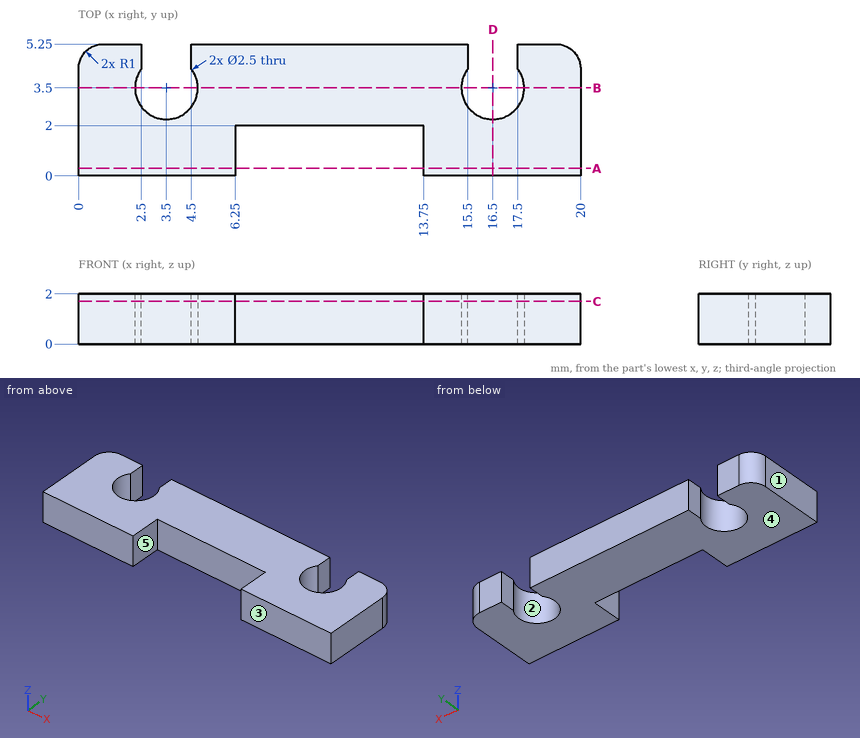
Answer from the drawing. Dimensions are ordinates in mm from the lowest x, y and z of the part. A direction names the side the tool comes from. Round coordinates to 2 decimals unless told otherwise and drop trailing zeros. Order: outer loops, then holes, each group sorted by start corner. A loop starts at its lowest first (then second) coordinate and runs counter-clockwise, first axis right, second up.
1) For the marked faces 4 and 5, determine the directions among +Z, -Z, +X, -X, +Y, -Y from which every point of the face is accessible in a straight line to the end or side of a thin tool.
2) The part is cut by section D-D on x = 16.5. Write down the section's boundary in (y, z).
3) The part is cut by section C-C on z = 1.7. Write down the section's boundary in (x, y).
4) Flat-ended cylindrical pins translate along their axes: pin 1 (0.5 mm diameter, centred on y = 5, z = 0.5, fed in from +X); pin 2 (1.1 mm diameter, centred on y = 5, z = 0.5, fed in from -X). Find the tip coordinate at first contact, or state that the pin passes through.
5) The mould has two halves that part along Y. Classify the marked faces 1, 2 and 3: released by +Y, released by -Y, zero draft, split by the parting line, or undercut.
6) Straight lines are drawn through the part: L1, parallel to X at y = 3.5, z = 1.1; L2, parallel to X at y = 0.3, z = 1; L3, parallel to X at y = 2.5, z = 0.1. For each, find the intervals that lie inside material, in ascending order.
7) The part is cut by section B-B on y = 3.5. Write down the section's boundary in (x, z).
8) The part is cut by section A-A on y = 0.3. Write down the section's boundary in (x, z).
Resolved:
1. face 4: -Z, +X, -X, +Y, -Y
1. face 5: +Z, -Z, -Y
2. outline: (0, 0) - (2.25, 0) - (2.25, 2) - (0, 2) - close
3. outline: (0, 0) - (6.25, 0) - (6.25, 2) - (13.75, 2) - (13.75, 0) - (20, 0) - (20, 4.25) arc R1 ccw to (19, 5.25) - (17.5, 5.25) - (17.5, 4.25) arc R1.25 cw (long way) to (15.5, 4.25) - (15.5, 5.25) - (4.5, 5.25) - (4.5, 4.25) arc R1.25 cw (long way) to (2.5, 4.25) - (2.5, 5.25) - (1, 5.25) arc R1 ccw to (0, 4.25) - close
4. pin 1: stops at x = 19.87
4. pin 2: stops at x = 0.02
5. face 1: zero draft
5. face 2: undercut
5. face 3: released by -Y
6. L1: x = 0 to 2.25, 4.75 to 15.25, 17.75 to 20
6. L2: x = 0 to 6.25, 13.75 to 20
6. L3: x = 0 to 2.75, 4.25 to 15.75, 17.25 to 20
7. outline: (0, 0) - (2.25, 0) - (2.25, 2) - (0, 2) - close; (4.75, 0) - (15.25, 0) - (15.25, 2) - (4.75, 2) - close; (17.75, 0) - (20, 0) - (20, 2) - (17.75, 2) - close
8. outline: (0, 0) - (6.25, 0) - (6.25, 2) - (0, 2) - close; (13.75, 0) - (20, 0) - (20, 2) - (13.75, 2) - close
